```python
from build123d import *

# Parameters (mm, degrees)
PADR_OCIRCULAR1_COUNT = 4
FILETE1_R             = 0.5


with BuildPart() as part:
    # Esboço1 → Revolução1 (revolve)
    with BuildSketch(Plane(origin=(0, 0, 0), x_dir=(0, 0, -1), z_dir=(-1, 0, 0)), mode=Mode.PRIVATE) as revolu_o1_sk:
        Polygon((0, 3), (0, 4.25), (-0.5, 4.25), (-0.5, 4.75), (0, 4.75), (0, 5.5), (-0.5, 5.5), (-0.5, 6), (0, 6), (0, 14), (-5, 14), (-5, 6), (-19, 6), (-19, 4.75), (-18.5, 4.75), (-18.5, 4.25), (-19, 4.25), (-19, 3), align=None)
    revolve(revolu_o1_sk.sketch.rotate(Axis((0, 0, 0), (0, 0, 1)), 270), axis=Axis((0, 0, 0), (0, 0, 1)))  # turned: the seam where the file's is

    # Esboço5 → Corte-Revolução1 (revolve, cut)
    with BuildSketch(Plane(origin=(0, 0, 0), x_dir=(0, 0, -1), z_dir=(1, 0, 0)), mode=Mode.PRIVATE) as corte_revolu_o1_sk:
        Polygon((0, 13), (-3.1, 13), (-3.1, 11.75), (-5, 11.75), (-5, 10), (0, 10), align=None)
    corte_revolu_o1 = revolve(corte_revolu_o1_sk.sketch.rotate(Axis((0, 10, 0), (0, 0, -1)), 90), axis=Axis((0, 10, 0), (0, 0, -1)), mode=Mode.SUBTRACT)  # turned: the seam where the file's is

    # PadrãoCircular1: Corte-Revolução1 ×4 about axis
    padr_ocircular1_axis = Axis((0, 0, 0), (0, 0, 1))
    for i in range(1, PADR_OCIRCULAR1_COUNT):
        add(corte_revolu_o1.rotate(padr_ocircular1_axis, i * 360 / PADR_OCIRCULAR1_COUNT), mode=Mode.SUBTRACT)

    # Filete1
    filete1_edges = [part.edges().sort_by_distance(p)[0] for p in [
        (6, 0, 19),
        (14, 0, 5),
        (14, 0, 0),
    ]]
    fillet(filete1_edges, radius=FILETE1_R)


solid = part.part
```
Design review of the part built by this model. Coordinates are the model's own, in mm. A direction names the side the tool comes from. Coordinates: 2 decimals unless noted, no trailing zeros. Order: outer loops, then holes, each group sorted by start corner. A loop starts at its lowest first (then second) coordinate and runs counter-clockwise, first axis right, second up. Notation, with made-up numbers: (8, 41.5) -> (41, 41.5) arc R29 cw to (41, 63.5) -> close; hole circle Ø11 at (19.25, -30). An arc over 180 degrees is marked (long way). One line per item, written item: value. Start each with the question number.
Q1. Tool access review of faces 1 (the cylindrical face through (-2.86, -0.9, 9.37)), 2 (the flat face through (-6, 3, 5)), 3 (the flat face through (0, -12, 3.1)): name each direction out of +Z, -Z, +X, -X, +Y, -Y from which nothing blocks a thin tool from reaching the whole face with its end or side.
Q2. Insertion check: pin 1 Ø1.8 at (x, y) = (0.5, 8.5) entering from -Z; pin 2 Ø4.5 at (x, y) = (0, 10) entering from +Z; pin 3 Ø10 at (x, z) = (-7.5, 4) entering from -Y (3 decimals). Each pin has a flat end and moves straight along its axis. Give the tip position at first contact, or say it passes through.
Q3. Take a section at C-C, the plane z = 15. State the section outline as (x, y) points, then the cut area to 3 significant figures.
Q4. Take a section at A-A, the plane y = 0. Give the number of separate pieces and of enclosed holes in the cut face, then the cut area to 3 significant figures.
Q5. For probe 1 along Y at (x, z) = (0, 4.05); probe 2 along Y at (x, z) = (0, 2); probe 3 along Z at (x, y) = (7, -10.75), list the stretches that pass through material, from the lowest coordinate up.
Q6. Mouldability with a two-part tool opening along X and no side actions: class faces 4 (the cylindrical face through (3.03, 13.67, 2.53)), 5 (the flat face through (5, 0, 19)), 6 (the flat face through (-12, 0, 3.1)) as pulls with the +X half, pulls with the -X half, needs draft (parallel to the pull), parting line crosses it, or undercut.
Values follow:
1. face 1: +Z, -Z
1. face 2: +Z
1. face 3: -Z
2. pin 1: stops at z = 3.1
2. pin 2: stops at z = 5
2. pin 3: stops at y = -13.775
3. outline: circle Ø12 at (0, 0); hole circle Ø6 at (0, 0)
3. area: 84.8 mm2
4. separate pieces: 4
4. enclosed holes: 0
4. area: 142 mm2
5. probe 1: y = -14 to -11.75, -8.25 to -3, 3 to 8.25, 11.75 to 14
5. probe 2: y = -14 to -13, -7 to -3, 3 to 7, 13 to 14
5. probe 3: z = 0 to 5
6. face 4: parting line crosses it
6. face 5: needs draft
6. face 6: undercut
